The model under review builds one solid part; all positions refer to its coordinate system, in mm. A direction names the side the tool comes from. Give positions to 0.01 mm unless a question says otherwise; leave off trailing zeros. Loops run counter-clockwise (first coordinate to the right, second up) from the corner with the lowest first, then second, coordinate; pieces in that order, holes last. Notation, with made-up numbers: M -30.75,-38 L 20.25,-38 A19 ccw 20.25,-6 Z; hole C 71,87 d7. An arc over 180 degrees is marked long. Return JSON: item names as keys, results as strings.
Autodesk Inventor part; units mm, degrees
ref_plane "YZ Plane" through (0, 0, 0) normal (1, 0, 0) x (0, 1, 0)
ref_plane "XZ Plane" through (0, 0, 0) normal (0, 1, 0) x (-1, 0, 0)
ref_plane "XY Plane" through (0, 0, 0) normal (0, 0, 1) x (1, 0, 0)
ref_plane "Work Plane1" through (-2.4672, -28.2462, -31.996) normal (1, 0, 0) x (0, 1, 0)
sketch "Sketch1" plane through (-2.4672, -28.2462, -31.996) normal (1, 0, 0) x (0, 1, 0)
  line L0 (0, 16.54) -> (22, 16.54)
  line L1 (22, 16.54) -> (22, -16.54)
  line L2 (22, -16.54) -> (0, -16.54)
  line L3 (0, -16.54) -> (0, 16.54)
  line L4 (0, -14) -> (0, 14)
  line L5 (0, 13) -> (22, 13) construction
  line L6 (0, -13) -> (22, -13) construction
  line L7 (22, -14) -> (22, 14)
  line L8 (22, 0) -> (0, 0) construction
  point P0 (28.2462, 31.996)
  dimension "d3" = 33.08
extrude "Extrusion1" add sketch "Sketch1" along normal blind 28.575 and the other way blind 15.875
sketch "Sketch5" plane through (-18.3422, -6.2462, -15.456) normal (0, 1, 0) x (1, 0, 0)
  circle A0 centre (15.875, 16.54) radius 4.5
  circle A1 centre (15.875, 16.54) radius 14
  circle A2 centre (15.875, 16.54) radius 14.254
  point P0 (18.3422, -15.456)
  dimension "d9" = 0.254
extrude "Extrusion2" cut sketch "Sketch5" against normal through all contours A0 | A1 | A2
sketch "Sketch6" plane through (-18.3422, -6.2462, -15.456) normal (0, 1, 0) x (1, 0, 0)
  circle A0 centre (15.875, 16.54) radius 14.254
  line L0 (0, 0) -> (44.45, 0)
  line L1 (44.45, 33.08) -> (44.45, 0)
  line L2 (0, 33.08) -> (44.45, 33.08)
  line L3 (0, 0) -> (0, 33.08)
  line L4 (44.45, 9.301) -> (41.91, 8.3485)
  line L5 (41.91, 8.3485) -> (41.91, 17.8735)
  line L6 (41.91, 17.8735) -> (44.45, 16.921)
  line L7 (44.45, 21.366) -> (41.91, 20.4135)
  line L8 (41.91, 20.4135) -> (41.91, 29.9385)
  line L9 (41.91, 29.9385) -> (44.45, 28.986)
  line L10 (0, 0) -> (0, 33.08)
  line L11 (0, 16.54) -> (44.6434, 16.54) construction
  point P0 (18.3422, -15.456)
  point P1 (41.91, 25.176)
  point P2 (41.91, 13.111)
  dimension "d12" = 9.525
  dimension "d13" = 7.62
  dimension "d14" = 7.62
  dimension "d15" = 2.54
  dimension "d61" = 8.636
  dimension "d62" = 12.065
extrude "Extrusion3" cut sketch "Sketch6" against normal through all contours L4 L5 L6 L1 | L1 L7 L8 L9
sketch "Sketch7" plane through (-18.3422, -28.2462, -15.456) normal (0, -1, 0) x (1, 0, 0)
  circle A0 centre (4.335, -28.08) radius 1.524
  circle A1 centre (4.335, -5) radius 1.524
  circle A2 centre (27.415, -5) radius 1.524
  circle A3 centre (27.415, -28.08) radius 1.524
  line L0 (3.2574, -29.1576) -> (2.1797, -28.08)
  line L1 (2.1797, -28.08) -> (3.2574, -27.0024)
  line L2 (44.45, -28.986) -> (41.91, -29.9385)
  line L3 (41.91, -29.9385) -> (41.91, -20.4135)
  line L4 (41.91, -20.4135) -> (44.45, -21.366)
  line L5 (44.45, -16.921) -> (44.45, -21.366)
  line L6 (44.45, -16.921) -> (41.91, -17.8735)
  line L7 (41.91, -17.8735) -> (41.91, -8.3485)
  line L8 (41.91, -8.3485) -> (44.45, -9.301)
  line L9 (44.45, 0) -> (44.45, -9.301)
  line L10 (44.45, 0) -> (0, 0)
  line L11 (0, -33.08) -> (0, 0)
  line L12 (0, -33.08) -> (44.45, -33.08)
  line L13 (44.45, -28.986) -> (44.45, -33.08)
  circle A4 centre (15.875, -16.54) radius 14.254
  line L14 (3.2574, -6.0776) -> (2.1797, -5)
  line L15 (2.1797, -5) -> (3.2574, -3.9224)
  line L16 (26.3374, -6.0776) -> (25.2597, -5)
  line L17 (25.2597, -5) -> (26.3374, -3.9224)
  line L18 (26.3374, -29.1576) -> (25.2597, -28.08)
  line L19 (25.2597, -28.08) -> (26.3374, -27.0024)
  point P0 (18.3422, 15.456)
extrude "Extrusion4" cut sketch "Sketch7" against normal blind 3.175 contours A0 | A0 L0 L1 | A1 | A1 L14 L15 | A2 | A2 L16 L17 | A3 | A3 L18 L19
fillet "Fillet1" radius 3.175 2 edges at (-18.3422, -17.2462, -48.536) (-18.3422, -17.2462, -15.456)
sketch "Sketch8" plane through (23.5678, -6.2462, -23.8045) normal (0, 1, 0) x (1, 0, 0)
  line L0 (5.715, -17.081) -> (5.715, -4.381)
  line L1 (5.715, -4.381) -> (-14.605, -17.081) construction
  line L2 (-14.605, -17.081) -> (5.715, -17.081)
  line L3 (-38.735, -8.3485) -> (2.54, -8.3485)
  line L4 (2.54, 0.9525) -> (2.54, -8.3485)
  line L5 (-16.2877, -14.3886) -> (4.0323, -1.6886)
  line L6 (-14.605, -17.081) -> (-16.2877, -14.3886)
  line L7 (5.715, -4.381) -> (4.0323, -1.6886)
  dimension "d26" = 20.32
  dimension "d27" = 12.7
  dimension "d28" = 8.7325
  dimension "d29" = 3.175
  dimension "d30" = 3.175
extrude "Extrusion5" cut sketch "Sketch8" along normal through all both and the other way through all
sketch "Sketch11" plane through (23.5678, -6.2462, -23.8045) normal (0, 1, 0) x (1, 0, 0)
  line L0 (2.54, 20.6375) -> (2.54, 24.7315)
  line L1 (2.54, 24.7315) -> (-10.6582, 32.3515)
  line L2 (-10.6582, 32.3515) -> (-18.2782, 32.3515)
  line L3 (-18.2782, 32.3515) -> (-18.2782, 24.7315)
  circle A0 centre (-26.035, 8.1915) radius 14.254
  line L4 (-6.6235, -8.3485) -> (2.54, -2.6213)
  line L5 (2.54, 0.9525) -> (2.54, -2.6213)
  line L6 (2.54, 0.9525) -> (0, 0)
  line L7 (0, 0) -> (0, 9.525)
  line L8 (0, 9.525) -> (2.54, 8.5725)
  line L9 (2.54, 13.0175) -> (2.54, 8.5725)
  line L10 (2.54, 13.0175) -> (0, 12.065)
  line L11 (0, 12.065) -> (0, 21.59)
  line L12 (0, 21.59) -> (2.54, 20.6375)
  line L13 (2.54, 24.7315) -> (2.54, 20.6375)
  line L14 (-38.735, 24.7315) -> (2.54, 24.7315)
  arc A1 (-38.735, 24.7315) -> (-41.91, 21.5565) centre (-38.735, 21.5565) ccw
  line L15 (-41.91, -5.1735) -> (-41.91, 21.5565)
  arc A2 (-41.91, -5.1735) -> (-38.735, -8.3485) centre (-38.735, -5.1735) ccw
  line L16 (-38.735, -8.3485) -> (-6.6235, -8.3485)
  circle A3 centre (-14.4682, 28.5415) radius 1.5875
  point P0 (-23.5678, -23.8045)
  point P1 (2.54, 24.7315)
  point P2 (-41.91, 8.1915)
  dimension "d42" = 120
  dimension "d43" = 7.62
  dimension "d45" = 7.62
  dimension "d46" = 3.175
  dimension "d47" = 3.81
  dimension "d48" = 3.81
  dimension "d53" = 20.35
  dimension "d63" = 11.5668
extrude "Extrusion7" add sketch "Sketch11" against normal blind 3.175 contours L14 L3 L2 L1 | A3
fillet "Fillet2" radius 3.175 1 edges at (5.2896, -7.8337, -56.156)
fillet "Fillet3" radius 3.175 1 edges at (5.2896, -7.8337, -48.536)
hole "Hole2" at (9.0996, -6.2462, -52.346) direction (0, -1, 0) diameter 4 depth 3.175
equation "\"d45\" = d43"
equation "\"d47\" = 0.5 * d43"
equation "\"d48\" = 0.5 * d43"
properties part number "Brushless Motor Seat_3DPrint"
1) Wall thickness on L1, parallel to X at y = -10.25, z = -32; L2, parallel to Z at x = 7, y = -26.75; L3, parallel to X at y = -21.25, z = -21: over which ranges is each line inside the solid? List them lowest first. Write a range as from..to.
From the geometry:
{"L1": "-18.34..-16.72, 11.79..23.57", "L2": "-48.54..-43.62, -43.45..-42.65, -21.34..-20.54, -20.37..-15.46", "L3": "-18.34..-11.54, 6.6..25.81"}
2) Consider section A-A on x = 0. Write out the cut boundary in (y, z), then the cut area to 3 significant figures.
From the geometry:
{"outline": "M -28.25,-48.54 L -6.25,-48.54 L -6.25,-46.03 L -28.25,-46.03 Z; M -28.25,-17.96 L -6.25,-17.96 L -6.25,-15.46 L -28.25,-15.46 Z", "area": "110 mm²"}
3) Consider section C-C on y = -25.75. Count the separate pieces of the cut face and the enclosed holes in it, then the cut area to 3 significant figures.
From the geometry:
{"separate pieces": "1", "enclosed holes": "5", "area": "727 mm²"}
4) Consider section B-B on z = -34. Write out the cut boundary in (x, y), then the cut area to 3 significant figures.
From the geometry:
{"outline": "M -18.34,-28.25 L -16.58,-28.25 L -16.58,-6.25 L -18.34,-6.25 Z; M 11.65,-28.25 L 26.11,-28.25 L 26.11,-6.25 L 11.65,-6.25 Z", "area": "357 mm²"}
5) Insertion check: pin 1 (3.5 mm diameter, centred on x = -14, z = -44, fed in from -Y); pin 2 (11 mm diameter, centred on x = -4, y = -17, fed in from -Z); pin 3 (6.5 mm diameter, centred on x = 9.1, z = -52.35, fed in from -Y); pin 4 (1.5 mm diameter, centred on x = 8.5, z = -20, fed in from -Y). Each pin has a flat end and moves straight along its axis. Give the tip position at first contact, or say it passes through.
From the geometry:
{"pin 1": "y = -28.25", "pin 2": "z = -48.54", "pin 3": "y = -9.42", "pin 4": "y = -25.07"}
6) The part is to be moulded in two halves that separate along X. For faces 1 (the face through (11, -8, -56.156)), 2 (the face through (7.449, -26.681, -19.925)), 3 (the face through (5.29, -8, -52)), say which applies: released by +X, released by -X, zero draft, split by the parting line, or undercut.
From the geometry:
{"face 1": "zero draft", "face 2": "undercut", "face 3": "released by -X"}
7) Tool access review of faces 4 (the face through (-12.484, -26.681, -20.506)), 5 (the face through (21.46, -17.4, -18.28)), 6 (the face through (23.568, -17, -41)): name each direction out of +Z, -Z, +X, -X, +Y, -Y from which nothing blocks a thin tool from reaching the whole face with its end or side.
From the geometry:
{"face 4": "-Y", "face 5": "+Z, +X, +Y, -Y", "face 6": "+Y, -Y"}
